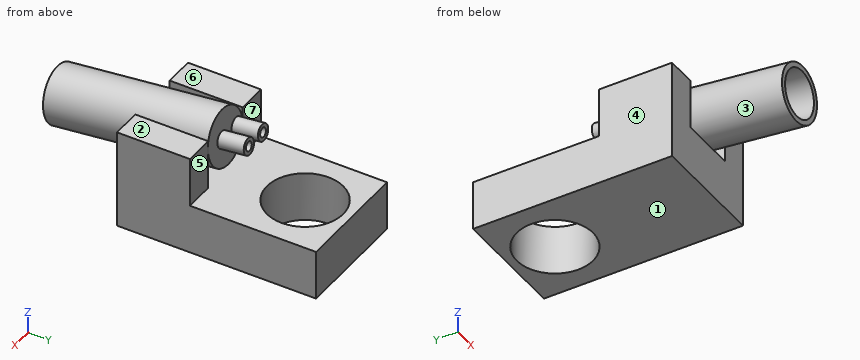
from build123d import *

# Parameters (mm, degrees)
CYLINDER010_R          = 11.5
CYLINDER010_DEPTH      = 20
BOX_W                  = 35
BOX_H                  = 60
BOX_DEPTH              = 15
BOX002_W               = 9
BOX002_H               = 22
BOX002_DEPTH           = 15
BOX001_W               = 9
BOX001_H               = 22
BOX001_DEPTH           = 15
CYLINDER009_R          = 1.4
CYLINDER009_DEPTH      = 50
CYLINDER008_R          = 2.5
CYLINDER008_DEPTH      = 12
CYLINDER007_R          = 1.4
CYLINDER007_DEPTH      = 50
CYLINDER006_R          = 2.5
CYLINDER006_DEPTH      = 12
CYLINDER005_R          = 3
CYLINDER005_DEPTH      = 60
CYLINDER004_R          = 4
CYLINDER004_DEPTH      = 40
CYLINDER002_R          = 7
CYLINDER002_DEPTH      = 46
CYLINDER_R             = 8.5
CYLINDER_DEPTH         = 50
CUT004_PLACEMENT_ANGLE = 6.4


with BuildPart() as cylinder010:
    # Cylinder010 → Cylinder010 (new body)
    with BuildSketch(Plane(origin=(17.5, 46, -2), x_dir=(1, 0, 0), z_dir=(0, 0, 1))):
        Circle(CYLINDER010_R)
    extrude(amount=CYLINDER010_DEPTH)


with BuildPart() as cut:
    # Box → Box (new body)
    with BuildSketch(Plane.XY):
        with Locations((17.5, 30)):
            Rectangle(BOX_W, BOX_H)
    extrude(amount=BOX_DEPTH)

    # Cut: cut Cylinder010
    add(cylinder010.part, mode=Mode.SUBTRACT)


with BuildPart() as cube002:
    # Box002 → Box002 (new body)
    with BuildSketch(Plane(origin=(26, 0, 15), x_dir=(1, 0, 0), z_dir=(0, 0, 1))):
        with Locations((4.5, 11)):
            Rectangle(BOX002_W, BOX002_H)
    extrude(amount=BOX002_DEPTH)


with BuildPart() as cube001:
    # Box001 → Box001 (new body)
    with BuildSketch(Plane.XY.offset(15)):
        with Locations((4.5, 11)):
            Rectangle(BOX001_W, BOX001_H)
    extrude(amount=BOX001_DEPTH)


with BuildPart() as cylinder009:
    # Cylinder009 → Cylinder009 (new body)
    with BuildSketch(Plane(origin=(11.9, 44, 26), x_dir=(1, 0, 0), z_dir=(0, -1, 0))):
        Circle(CYLINDER009_R)
    extrude(amount=CYLINDER009_DEPTH)


with BuildPart() as cylinder008:
    # Cylinder008 → Cylinder008 (new body)
    with BuildSketch(Plane(origin=(11.9, 30, 26), x_dir=(1, 0, 0), z_dir=(0, -1, 0))):
        Circle(CYLINDER008_R)
    extrude(amount=CYLINDER008_DEPTH)


with BuildPart() as cylinder007:
    # Cylinder007 → Cylinder007 (new body)
    with BuildSketch(Plane(origin=(18.9, 45, 26), x_dir=(1, 0, 0), z_dir=(0, -1, 0))):
        Circle(CYLINDER007_R)
    extrude(amount=CYLINDER007_DEPTH)


with BuildPart() as cylinder006:
    # Cylinder006 → Cylinder006 (new body)
    with BuildSketch(Plane(origin=(18.9, 30, 26), x_dir=(1, 0, 0), z_dir=(0, -1, 0))):
        Circle(CYLINDER006_R)
    extrude(amount=CYLINDER006_DEPTH)


with BuildPart() as cylinder005:
    # Cylinder005 → Cylinder005 (new body)
    with BuildSketch(Plane(origin=(17.5, 18, 26), x_dir=(1, 0, 0), z_dir=(0, -1, 0))):
        Circle(CYLINDER005_R)
    extrude(amount=CYLINDER005_DEPTH)


with BuildPart() as cut002:
    # Cylinder004 → Cylinder004 (new body)
    with BuildSketch(Plane(origin=(17.5, 22, 26), x_dir=(1, 0, 0), z_dir=(0, -1, 0))):
        Circle(CYLINDER004_R)
    extrude(amount=CYLINDER004_DEPTH)

    # Cut002: cut Cylinder005
    add(cylinder005.part, mode=Mode.SUBTRACT)


with BuildPart() as cylinder002:
    # Cylinder002 → Cylinder002 (new body)
    with BuildSketch(Plane(origin=(17.5, 18, 26), x_dir=(1, 0, 0), z_dir=(0, -1, 0))):
        Circle(CYLINDER002_R)
    extrude(amount=CYLINDER002_DEPTH)


with BuildPart() as fusion004:
    # Cylinder → Cylinder (new body)
    with BuildSketch(Plane(origin=(17.5, 22, 26), x_dir=(1, 0, 0), z_dir=(0, -1, 0))):
        Circle(CYLINDER_R)
    extrude(amount=CYLINDER_DEPTH)

    # Cut001: cut Cylinder002
    add(cylinder002.part, mode=Mode.SUBTRACT)

    # Fusion: union Cut002
    add(cut002.part)

    # Fusion001: union Cylinder006
    add(cylinder006.part)

    # Cut003: cut Cylinder007
    add(cylinder007.part, mode=Mode.SUBTRACT)

    # Fusion002: union Cylinder008
    add(cylinder008.part)

    # Cut004: cut Cylinder009
    add(cylinder009.part, mode=Mode.SUBTRACT)


with BuildPart() as fusion004_1:
    # Cut004 placement: moved
    add(fusion004.part.moved(Location((0, 3, -2.3))).rotate(Axis((0, 3, -2.3), (1, 0, 0)), CUT004_PLACEMENT_ANGLE))

    # Fusion003: union Cube002, Cube001
    add(cube002.part)
    add(cube001.part)

    # Fusion004: union Cut
    add(cut.part)


solid = fusion004_1.part
Design review of the part built by this model. Coordinates are the model's own, in mm. Face numbers are marked on the shaded views. A direction names the side the tool comes from. Give positions to 0.01 mm unless a question says otherwise; leave off trailing zeros. Write each loop counter-clockwise with the first axis right and the second up, starting at its lowest first coordinate (ties: lowest second). Pieces come first, ordered by that corner, then holes. Notation, with made-up numbers: M 48,-17 L 92,-17 A15 cw 92,-12 Z; hole C 0.5,20.5 d10. An arc over 180 degrees is marked long. Return JSON: item names as keys, results as strings. Group by question number.
Item 1: Clearance check with flat-ended pins moving along their axes: pin 1 Ø4 at (x, z) = (13.5, 27.5) entering from +Y; pin 2 Ø15 at (x, z) = (22, 10.5) entering from -Y; pin 3 Ø4.5 at (x, y) = (5, 12) entering from +Z. State where each tip first meets the part, or that it passes through.
Item 2: The part is to be moulded in two halves that separate along Z. For the marked faces 1, 2, 3 and 4, say which applies: pulls with the +Z half, pulls with the -Z half, needs draft (parallel to the pull), parting line crosses it, or undercut.
Item 3: Take a section at C-C (x = 7.5). Give the boundary of the cut face in (y, z), plus the area to 3 significant figures.
Item 4: Take a section at B-B (x = 32.5). Give the boundary of the cut face in (y, z).
Item 5: Take a section at D-D (y = 37). Give the boundary of the cut face in (x, z).
Item 6: Tool access review of the marked faces 5, 6 and 7: name each direction out of +Z, -Z, +X, -X, +Y, -Y from which nothing blocks a thin tool from reaching the whole face with its end or side.
Item 7: Take a section at A-A (y = 46). Give the boundary of the cut face in (x, z).
Item 8: Wall thickness on line 1 along X through (y, z) = (46, 4); line 2 along Y through (x, z) = (17.5, 10); line 3 along Z through (x, y) = (14, -16.5): over which ranges is each line inside the solid? List them lowest first.
Return value:
{
 "1": {"pin 1": "stops at y = 30.07", "pin 2": "stops at y = -27.42", "pin 3": "stops at z = 30"},
 "2": {"face 1": "pulls with the -Z half", "face 2": "pulls with the +Z half", "face 3": "undercut", "face 4": "needs draft"},
 "3": {"outline": "M 0,0 L 40.32,0 L 40.32,15 L 22,15 L 22,30 L 0,30 Z; M 51.68,0 L 60,0 L 60,15 L 51.68,15 Z", "area": "1,060 mm2"},
 "4": {"outline": "M 0,0 L 60,0 L 60,15 L 22,15 L 22,30 L 0,30 Z"},
 "5": {"outline": "M 0,0 L 10.34,0 L 10.34,15 L 0,15 Z; M 24.66,0 L 35,0 L 35,15 L 24.66,15 Z"},
 "6": {"face 5": "+Z, +X, +Y", "face 6": "+Z, -X, +Y, -Y", "face 7": "+Z, -X, +Y"},
 "7": {"outline": "M 0,0 L 6,0 L 6,15 L 0,15 Z; M 29,0 L 35,0 L 35,15 L 29,15 Z"},
 "8": {"line 1": "x = 0 to 6, 29 to 35", "line 2": "y = 0 to 34.5, 57.5 to 60", "line 3": "z = 13.88 to 15.58, 19.73 to 23.62, 27.78 to 29.47"}
}
